Build history of the part. All positions in model axes, mm. Face numbers are marked on the shaded views. Coordinates: 2 decimals unless noted, no trailing zeros. Write each loop counter-clockwise with the first axis right and the second up, starting at its lowest first coordinate (ties: lowest second). Pieces come first, ordered by that corner, then holes. Notation, with made-up numbers: (-10.5, 46.25) -> (44.5, 46.25) arc R26 cw to (44.5, 76.25) -> close; hole circle Ø7 at (31, 47.5). An arc over 180 degrees is marked (long way). Write each question's results on one line, items separated by ' | '. Start each with the question number.
Q1. Saw through at C-C on y = 0. Give the cut face in (x, z).
Q2. Two-plate mould, pull along X, no slides. Class the marked faces 1, 2 and 3: released by +X, released by -X, zero draft, split by the parting line, or undercut.
Q3. Drill centre lines: line 1 (Y direction, x = 0.6, z = -1.5); line 2 (X direction, y = -0.05, z = -9.25); line 3 (Y direction, x = 0.15, z = -9.5). Where is each one in solid material? Low to high.
Q4. Saw through at A-A on z = -5. Give the cut face in (x, y).
Q5. Saw through at B-B on x = 0.9. Give the cut face in (y, z), and give its area (3 significant figures).
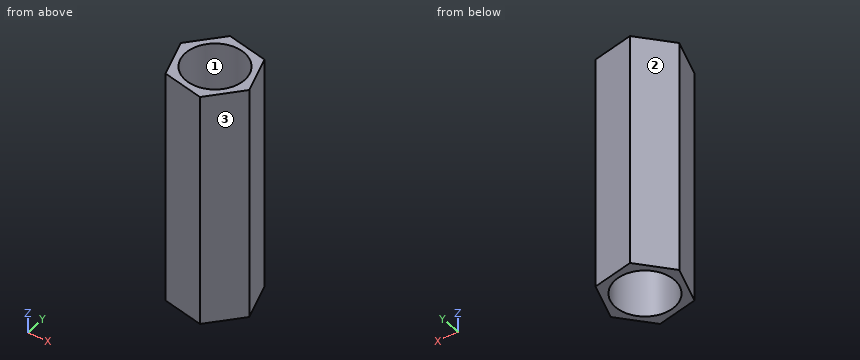
from build123d import *

# Parameters (mm, degrees)
EXTRUDE_1_DEPTH    = 10
HOLE_WIZARD_M3_1_D = 2.5


with BuildPart() as part:
    # 草图1 → 凸台-拉伸1 (new body)
    with BuildSketch(Plane.XY):
        Polygon((0.562771868, -1.638074426), (1.7, -0.331662479), (1.137228132, 1.306411947), (-0.562771868, 1.638074426), (-1.7, 0.331662479), (-1.137228132, -1.306411947), align=None)
    extrude(amount=-EXTRUDE_1_DEPTH)

    # M3 螺纹孔1 (through all)
    with Locations(Plane(origin=(0, 0, -10), x_dir=(-1, 0, 0), z_dir=(0, 0, -1))):
        with Locations((0, 0)):
            Hole(HOLE_WIZARD_M3_1_D / 2)


solid = part.part
Returned:
1) outline: (-1.59, -10) -> (-1.25, -10) -> (-1.25, 0) -> (-1.59, 0) -> close; (1.25, -10) -> (1.59, -10) -> (1.59, 0) -> (1.25, 0) -> close
2) face 1: undercut | face 2: released by -X | face 3: released by +X
3) line 1: y = -1.6 to -1.1, 1.1 to 1.41 | line 2: x = -1.57 to -1.25, 1.25 to 1.6 | line 3: y = -1.56 to -1.24, 1.24 to 1.5
4) outline: (-1.7, 0.33) -> (-1.14, -1.31) -> (0.56, -1.64) -> (1.7, -0.33) -> (1.14, 1.31) -> (-0.56, 1.64) -> close; hole circle Ø2.5 at (0, 0)
5) outline: (-1.25, -10) -> (-0.87, -10) -> (-0.87, 0) -> (-1.25, 0) -> close; (0.87, -10) -> (1.35, -10) -> (1.35, 0) -> (0.87, 0) -> close | area: 8.68 mm2
